```python
from build123d import *

# Parameters (mm, degrees)
F0_W     = 2
F0_H     = 80
F0_R     = 1.5
F0_W_2   = 120
F0_H_2   = 2
F0_H_3   = 40
F1_DEPTH = 20


with BuildPart() as f1:
    # F0 (on Top) → F1 (new body)
    with BuildSketch(Plane.XY):
        with Locations((69.537793, -4.311995)):
            Rectangle(F0_W, F0_H)
        Polygon((70.537793, -54.311995), (70.537793, -44.311995), (68.537793, -44.311995), (60.537793, -44.311995), (60.537793, -52.311995), (60.537793, -54.311995), align=None)
        with Locations((65.537793, -49.311995)):
            Circle(F0_R, mode=Mode.SUBTRACT)
        with Locations((0.537793, -53.311995)):
            Rectangle(F0_W_2, F0_H_2)
        with Locations((-68.462207, -24.311995)):
            Rectangle(F0_W, F0_H_3)
        Polygon((-67.462207, -44.311995), (-69.462207, -44.311995), (-69.462207, -54.311995), (-59.462207, -54.311995), (-59.462207, -52.311995), (-59.462207, -44.311995), align=None)
        with Locations((-64.462207, -49.311995)):
            Circle(F0_R, mode=Mode.SUBTRACT)
        with Locations((-68.462207, 15.688005)):
            Rectangle(F0_W, F0_H_3)
        Polygon((-59.462207, 45.688005), (-69.462207, 45.688005), (-69.462207, 35.688005), (-67.462207, 35.688005), (-59.462207, 35.688005), (-59.462207, 43.688005), align=None)
        with Locations((-64.462207, 40.688005)):
            Circle(F0_R, mode=Mode.SUBTRACT)
        with Locations((0.537793, 44.688005)):
            Rectangle(F0_W_2, F0_H_2)
        Polygon((70.537793, 45.688005), (60.537793, 45.688005), (60.537793, 43.688005), (60.537793, 35.688005), (68.537793, 35.688005), (70.537793, 35.688005), align=None)
        with Locations((65.537793, 40.688005)):
            Circle(F0_R, mode=Mode.SUBTRACT)
    extrude(amount=F1_DEPTH)


solid = f1.part
```
Design review of the part built by this model. Coordinates are the model's own, in mm. A direction names the side the tool comes from. Coordinates: 2 decimals unless noted, no trailing zeros. Order: outer loops, then holes, each group sorted by start corner. A loop starts at its lowest first (then second) coordinate and runs counter-clockwise, first axis right, second up. Notation, with made-up numbers: (73.25, -34.5) -> (95.25, -34.5) arc R18 ccw to (95.25, -2.5) -> close; hole circle Ø3 at (13.5, 12). An arc over 180 degrees is marked (long way). One line per item, written item: value. Start each with the question number.
Q1. For probe 1 along Y at (x, z) = (-62, 12); probe 2 along Y at (x, z) = (29, 17.5); probe 3 along X at (y, z) = (35, 4.5), list the stretches that pass through material, from the lowest coordinate up.
Q2. Tool access review of faces 1 (the flat face through (68.538, -5, 10)), 2 (the flat face through (0, 44, 0)): name each direction out of +Z, -Z, +X, -X, +Y, -Y from which nothing blocks a thin tool from reaching the whole face with its end or side.
Q3. Mouldability with a two-part tool opening along X and no side actions: class faces 3 (the flat face through (2, 45.688, 10)), 4 (the flat face through (70.538, -5, 10)), 5 (the flat face through (-64, 35.688, 10)) as pulls with the +X half, pulls with the -X half, needs draft (parallel to the pull), parting line crosses it, or undercut.
Q4. Take a section at B-B, the plane x = 13. State the section outline as (y, z) points.
Q5. Take a section at A-A, the plane y = -30. State the section outline as (x, z) points.
Q6. Take a section at C-C, the plane z = 1.75. State the section outline as (x, y) points.
Values follow:
1. probe 1: y = -54.31 to -44.31, 35.69 to 45.69
1. probe 2: y = -54.31 to -52.31, 43.69 to 45.69
1. probe 3: x = -69.46 to -67.46, 68.54 to 70.54
2. face 1: +Z, -Z
2. face 2: -Z, +X, -X, +Y, -Y
3. face 3: needs draft
3. face 4: pulls with the +X half
3. face 5: undercut
4. outline: (-54.31, 0) -> (-52.31, 0) -> (-52.31, 20) -> (-54.31, 20) -> close; (43.69, 0) -> (45.69, 0) -> (45.69, 20) -> (43.69, 20) -> close
5. outline: (-69.46, 0) -> (-67.46, 0) -> (-67.46, 20) -> (-69.46, 20) -> close; (68.54, 0) -> (70.54, 0) -> (70.54, 20) -> (68.54, 20) -> close
6. outline: (-69.46, -54.31) -> (70.54, -54.31) -> (70.54, 45.69) -> (-69.46, 45.69) -> close; hole (-67.46, -44.31) -> (-59.46, -44.31) -> (-59.46, -52.31) -> (60.54, -52.31) -> (60.54, -44.31) -> (68.54, -44.31) -> (68.54, 35.69) -> (60.54, 35.69) -> (60.54, 43.69) -> (-59.46, 43.69) -> (-59.46, 35.69) -> (-67.46, 35.69) -> close; hole circle Ø3 at (-64.46, -49.31); hole circle Ø3 at (-64.46, 40.69); hole circle Ø3 at (65.54, -49.31); hole circle Ø3 at (65.54, 40.69)
